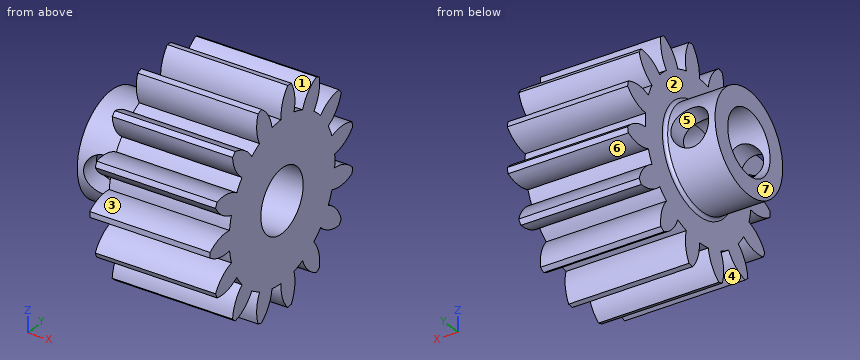
```python
from build123d import *

# Parameters (mm, degrees)
BASPROSKE_W                = 12.7
BASPROSKE_H                = 8.5
TOOTHCUT_DEPTH             = 18.486852204
TEETHCUTS_COUNT            = 15
TEETHCUTS_ANGLE            = 336
BORSKE_R                   = 0.4
BORE_DEPTH                 = 50.0000508
CORTAR_EXTRUIR1_START      = -3.18
CORTAR_EXTRUIR1_DEPTH      = 3.18
CROQUIS4_R                 = 2.5
CORTAR_EXTRUIR2_DEPTH      = 9.52
CROQUIS5_R                 = 4
CROQUIS5_R_2               = 2.5
SALIENTE_EXTRUIR1_DEPTH    = 4
CORTAR_EXTRUIR3_DEPTH      = 16.319316842
CORTAR_EXTRUIR3_DEPTH_BACK = 16.319316842
CROQUIS6_R                 = 1.5
REDONDEO2_R                = 0.25


with BuildPart() as part:
    # BasProSke → Base-Revolve (revolve)
    with BuildSketch(Plane(origin=(0, 0, 0), x_dir=(1, 0, 0), z_dir=(0, 1, 0)), mode=Mode.PRIVATE) as base_revolve_sk:
        with Locations((6.35, 4.25)):
            Rectangle(BASPROSKE_W, BASPROSKE_H)
    revolve(base_revolve_sk.sketch.rotate(Axis((-10, 0, 0), (1, 0, 0)), 180), axis=Axis((-10, 0, 0), (1, 0, 0)))

    # TooCutSke → ToothCut (cut, through all)
    with BuildSketch(Plane(origin=(0, 0, 0), x_dir=(0, 0, -1), z_dir=(1, 0, 0))):
        with BuildLine():
            ThreePointArc((0.531576138, 6.226349477), (0, 6.249), (-0.531576138, 6.226349477))
            ThreePointArc((-0.531576138, 6.226349477), (-0.830301624, 7.411024729), (-1.576608494, 8.378350125))
            ThreePointArc((-1.576608494, 8.378350125), (0, 8.5254), (1.576608494, 8.378350125))
            ThreePointArc((1.576608494, 8.378350125), (0.830301624, 7.411024729), (0.531576138, 6.226349477))
        make_face()
    toothcut = extrude(amount=TOOTHCUT_DEPTH, mode=Mode.SUBTRACT)

    # TeethCuts: ToothCut ×15 about axis
    teethcuts_axis = Axis((-10, 0, 0), (1, 0, 0))
    for i in range(1, TEETHCUTS_COUNT):
        add(toothcut.rotate(teethcuts_axis, i * TEETHCUTS_ANGLE / (TEETHCUTS_COUNT - 1)), mode=Mode.SUBTRACT)

    # BorSke → Bore (cut, symmetric)
    with BuildSketch(Plane(origin=(0, 0, 0), x_dir=(0, 0, -1), z_dir=(1, 0, 0))):
        with Locations(Location((0, 0, 0), (0, 0, 180))):
            Circle(BORSKE_R)
    extrude(amount=BORE_DEPTH, both=True, mode=Mode.SUBTRACT)

    # Croquis2 → Cortar-Extruir1 (cut)
    with BuildSketch(Plane(origin=(12.7, 0, 0), x_dir=(0, 0, -1), z_dir=(1, 0, 0)).offset(CORTAR_EXTRUIR1_START)):
        with BuildLine():
            ThreePointArc((-8.473551116, 0.670023493), (-7.441942771, 0.04560728), (-6.24780572, -0.122166634))
            ThreePointArc((-6.24780572, -0.122166634), (-6.214767324, -0.653198367), (-6.136676046, -1.179494851))
            ThreePointArc((-6.136676046, -1.179494851), (-7.26983618, -1.591877556), (-8.149077977, -2.417132211))
            ThreePointArc((-8.149077977, -2.417132211), (-8.083980389, -2.626644452), (-8.013497238, -2.834406818))
            ThreePointArc((-8.013497238, -2.834406818), (-6.817103167, -2.985246497), (-5.657964889, -2.652816299))
            ThreePointArc((-5.657964889, -2.652816299), (-5.411792748, -3.1245), (-5.126388751, -3.573533178))
            ThreePointArc((-5.126388751, -3.573533178), (-5.993850886, -4.411161274), (-6.461416928, -5.522688773))
            ThreePointArc((-6.461416928, -5.522688773), (-6.316731017, -5.687610154), (-6.167836888, -5.84874244))
            ThreePointArc((-6.167836888, -5.84874244), (-5.013524493, -5.499924035), (-4.089810528, -4.724769925))
            ThreePointArc((-4.089810528, -4.724769925), (-3.673070042, -5.055547198), (-3.229702268, -5.349675154))
            ThreePointArc((-3.229702268, -5.349675154), (-3.681474322, -6.467715134), (-3.656518192, -7.673322273))
            ThreePointArc((-3.656518192, -7.673322273), (-3.457261466, -7.76513639), (-3.255701506, -7.851777359))
            ThreePointArc((-3.255701506, -7.851777359), (-2.343061889, -7.063614742), (-1.814490772, -5.979767908))
            ThreePointArc((-1.814490772, -5.979767908), (-1.299240156, -6.112444357), (-0.774570923, -6.200809696))
            ThreePointArc((-0.774570923, -6.200809696), (-0.732537403, -7.405942289), (-0.219374243, -8.497168643))
            ThreePointArc((-0.219374243, -8.497168643), (0, -8.5), (0.219374243, -8.497168643))
            ThreePointArc((0.219374243, -8.497168643), (0.732537403, -7.405942289), (0.774570923, -6.200809696))
            ThreePointArc((0.774570923, -6.200809696), (1.299240156, -6.112444357), (1.814490772, -5.979767908))
            ThreePointArc((1.814490772, -5.979767908), (2.343061889, -7.063614742), (3.255701506, -7.851777359))
            ThreePointArc((3.255701506, -7.851777359), (3.457261466, -7.76513639), (3.656518192, -7.673322273))
            ThreePointArc((3.656518192, -7.673322273), (3.681474322, -6.467715134), (3.229702268, -5.349675154))
            ThreePointArc((3.229702268, -5.349675154), (3.673070042, -5.055547198), (4.089810528, -4.724769925))
            ThreePointArc((4.089810528, -4.724769925), (5.013524493, -5.499924035), (6.167836888, -5.84874244))
            ThreePointArc((6.167836888, -5.84874244), (6.316731017, -5.687610154), (6.461416928, -5.522688773))
            ThreePointArc((6.461416928, -5.522688773), (5.993850886, -4.411161274), (5.126388751, -3.573533178))
            ThreePointArc((5.126388751, -3.573533178), (5.411792748, -3.1245), (5.657964889, -2.652816299))
            ThreePointArc((5.657964889, -2.652816299), (6.817103167, -2.985246497), (8.013497238, -2.834406818))
            ThreePointArc((8.013497238, -2.834406818), (8.083980389, -2.626644452), (8.149077977, -2.417132211))
            ThreePointArc((8.149077977, -2.417132211), (7.26983618, -1.591877556), (6.136676046, -1.179494851))
            ThreePointArc((6.136676046, -1.179494851), (6.214767324, -0.653198367), (6.24780572, -0.122166634))
            ThreePointArc((6.24780572, -0.122166634), (7.441942771, 0.04560728), (8.473551116, 0.670023493))
            ThreePointArc((8.473551116, 0.670023493), (8.453436111, 0.888491938), (8.427689411, 1.106368468))
            ThreePointArc((8.427689411, 1.106368468), (7.288800753, 1.502656253), (6.085876303, 1.418488851))
            ThreePointArc((6.085876303, 1.418488851), (5.94315217, 1.931047198), (5.757344182, 2.429606752))
            ThreePointArc((5.757344182, 2.429606752), (6.780002862, 3.068575145), (7.468451026, 4.058600654))
            ThreePointArc((7.468451026, 4.058600654), (7.361215932, 4.25), (7.249076783, 4.438567989))
            ThreePointArc((7.249076783, 4.438567989), (6.04746546, 4.337367144), (4.982773259, 3.771202944))
            ThreePointArc((4.982773259, 3.771202944), (4.643912014, 4.181397159), (4.271385532, 4.561279057))
            ThreePointArc((4.271385532, 4.561279057), (4.945738865, 5.560958489), (5.171987905, 6.745408891))
            ThreePointArc((5.171987905, 6.745408891), (4.996174644, 6.876644452), (4.817032924, 7.003298781))
            ThreePointArc((4.817032924, 7.003298781), (3.760468449, 6.422107853), (3.018103451, 5.471841788))
            ThreePointArc((3.018103451, 5.471841788), (2.541697283, 5.708745565), (2.046865518, 5.904264776))
            ThreePointArc((2.046865518, 5.904264776), (2.256311686, 7.091801591), (1.981241089, 8.265874651))
            ThreePointArc((1.981241089, 8.265874651), (1.767249372, 8.314254606), (1.55208031, 8.357095591))
            ThreePointArc((1.55208031, 8.357095591), (0.823252281, 7.396407771), (0.531576138, 6.226349477))
            ThreePointArc((0.531576138, 6.226349477), (0, 6.249), (-0.531576138, 6.226349477))
            ThreePointArc((-0.531576138, 6.226349477), (-0.823252281, 7.396407771), (-1.55208031, 8.357095591))
            ThreePointArc((-1.55208031, 8.357095591), (-1.767249372, 8.314254606), (-1.981241089, 8.265874651))
            ThreePointArc((-1.981241089, 8.265874651), (-2.256311686, 7.091801591), (-2.046865518, 5.904264776))
            ThreePointArc((-2.046865518, 5.904264776), (-2.541697283, 5.708745565), (-3.018103451, 5.471841788))
            ThreePointArc((-3.018103451, 5.471841788), (-3.760468449, 6.422107853), (-4.817032924, 7.003298781))
            ThreePointArc((-4.817032924, 7.003298781), (-4.996174644, 6.876644452), (-5.171987905, 6.745408891))
            ThreePointArc((-5.171987905, 6.745408891), (-4.945738865, 5.560958489), (-4.271385532, 4.561279057))
            ThreePointArc((-4.271385532, 4.561279057), (-4.643912014, 4.181397159), (-4.982773259, 3.771202944))
            ThreePointArc((-4.982773259, 3.771202944), (-6.04746546, 4.337367144), (-7.249076783, 4.438567989))
            ThreePointArc((-7.249076783, 4.438567989), (-7.361215932, 4.25), (-7.468451026, 4.058600654))
            ThreePointArc((-7.468451026, 4.058600654), (-6.780002862, 3.068575145), (-5.757344182, 2.429606752))
            ThreePointArc((-5.757344182, 2.429606752), (-5.94315217, 1.931047198), (-6.085876303, 1.418488851))
            ThreePointArc((-6.085876303, 1.418488851), (-7.288800753, 1.502656253), (-8.427689411, 1.106368468))
            ThreePointArc((-8.427689411, 1.106368468), (-8.453436111, 0.888491938), (-8.473551116, 0.670023493))
        make_face()
    extrude(amount=CORTAR_EXTRUIR1_DEPTH, mode=Mode.SUBTRACT)

    # Croquis4 → Cortar-Extruir2 (cut)
    with BuildSketch(Plane(origin=(9.52, 0, 0), x_dir=(0, 0, -1), z_dir=(1, 0, 0))):
        Circle(CROQUIS4_R)
    extrude(amount=-CORTAR_EXTRUIR2_DEPTH, mode=Mode.SUBTRACT)

    # Croquis5 → Saliente-Extruir1 (add)
    with BuildSketch(Plane.ZY):
        with Locations(Location((0, 0, 0), (0, 0, 180))):
            Circle(CROQUIS5_R)
        with Locations(Location((0, 0, 0), (0, 0, 180))):
            Circle(CROQUIS5_R_2, mode=Mode.SUBTRACT)
    extrude(amount=SALIENTE_EXTRUIR1_DEPTH)

    # Croquis6 → Cortar-Extruir3 (cut, two sides: drawn at the far end of the back side and taken through both)
    with BuildSketch(Plane(origin=(0, 0, 0), x_dir=(1, 0, 0), z_dir=(0, 1, 0)).offset(-CORTAR_EXTRUIR3_DEPTH_BACK)):
        with Locations(Location((-2, 0, 0), (0, 0, 270))):
            Circle(CROQUIS6_R)
    extrude(amount=CORTAR_EXTRUIR3_DEPTH + CORTAR_EXTRUIR3_DEPTH_BACK, mode=Mode.SUBTRACT)

    # Redondeo2
    redondeo2_edges = [part.edges().sort_by_distance(p)[0] for p in [
        (0, 0, 4),
    ]]
    fillet(redondeo2_edges, radius=REDONDEO2_R)


solid = part.part
```
The model under review builds one solid part; all positions refer to its coordinate system, in mm. Face numbers are marked on the shaded views. A direction names the side the tool comes from. Give positions to 0.01 mm unless a question says otherwise; leave off trailing zeros. Write each loop counter-clockwise with the first axis right and the second up, starting at its lowest first coordinate (ties: lowest second). Pieces come first, ordered by that corner, then holes. Notation, with made-up numbers: M 82.25,37.25 L 111.25,37.25 A28 cw 111.25,76.25 Z; hole C 52.25,-33 d4. An arc over 180 degrees is marked long. Answer in a Markdown table with one row per item.
Item 1: For line 1 along X through (y, z) = (-3.1, 0); line 2 along Z through (x, y) = (2.25, 4); line 3 along Z through (x, y) = (-2, -3.15), list the stretches that pass through material, from the lowest coordinate up.
Check sheet entries:
| item | result |
|---|---|
| line 1 | -4 to -3.5, -0.5 to 9.52 |
| line 2 | -7.44 to -5.3, -4.8 to 4.8, 5.3 to 7.44 |
| line 3 | -2.47 to -1.5, 1.5 to 2.47 |
Item 2: Draft analysis for pull direction X (two halves, no side actions). For the marked faces 5, 6 and 7, state which applies: +X half, -X half, draft (parallel to the pull), parting line (faces both ways), or undercut.
Check sheet entries:
| item | result |
|---|---|
| face 5 | undercut |
| face 6 | draft |
| face 7 | -X half |
Item 3: Add section B-B on x = -2. Give the boundary of the cut face in (y, z), plus the area to 3 significant figures.
Check sheet entries:
| item | result |
|---|---|
| outline | M -3.71,-1.5 A4 ccw 3.71,-1.5 L 2,-1.5 A2.5 cw -2,-1.5 Z; M -3.71,1.5 L -2,1.5 A2.5 cw 2,1.5 L 3.71,1.5 A4 ccw Z |
| area | 21.2 mm2 |
Item 4: For P1, Ø2, axis at x = 4.5, z = 6, coming from the +Y side; P2, Ø1, axis at x = 0, y = -2.5, coming from the -Z side; P3, Ø3.5, axis at x = -2, z = 0, coming from the +Y side; P4, Ø2.5, axis at x = -2, z = 0, coming from the -Y side, all flat-tipped, find the tip position at first contact; note any pin that passes through.
Check sheet entries:
| item | result |
|---|---|
| P1 | y = 6.87 |
| P2 | z = -8.15 |
| P3 | y = 4 |
| P4 | through |
Item 5: Add section A-A on y = -6.75. Give the boundary of the cut face in (x, z), plus the area to 3 significant figures.
Check sheet entries:
| item | result |
|---|---|
| outline | M 0,-3.72 L 9.52,-3.72 L 9.52,-2.13 L 0,-2.13 Z; M 0,-0.82 L 9.52,-0.82 L 9.52,0.82 L 0,0.82 Z; M 0,2.13 L 9.52,2.13 L 9.52,3.72 L 0,3.72 Z |
| area | 45.8 mm2 |
Item 6: Tool access review of the marked faces 1, 2, 3 and 4: name each direction out of +Z, -Z, +X, -X, +Y, -Y from which nothing blocks a thin tool from reaching the whole face with its end or side.
Check sheet entries:
| item | result |
|---|---|
| face 1 | +Z, +X, -X |
| face 2 | -X |
| face 3 | +X, -X |
| face 4 | -Z, +X, -X |
Item 7: Add section C-C on y = 5.25. Give the boundary of the cut face in (x, z), plus the area to 3 significant figures.
Check sheet entries:
| item | result |
|---|---|
| outline | M 0,-4.8 L 9.52,-4.8 L 9.52,4.8 L 0,4.8 Z |
| area | 91.3 mm2 |
